CAD build for the part. Positions are in the model's coordinates, mm. Face numbers are marked on the shaded views. A direction names the side the tool comes from. Round coordinates to 2 decimals unless told otherwise and drop trailing zeros. Write each loop counter-clockwise with the first axis right and the second up, starting at its lowest first coordinate (ties: lowest second). Pieces come first, ordered by that corner, then holes. Notation, with made-up numbers: (7, 33) - (44, 33) arc R19 cw to (44, 55) - close; hole circle Ø11 at (36.25, 1). An arc over 180 degrees is marked (long way). Answer in a Markdown table with one row per item.
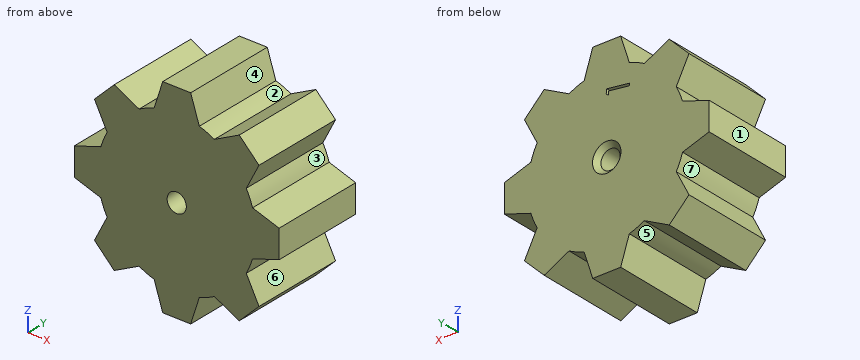
```python
from build123d import *

# Parameters (mm, degrees)
SKETCH1_R           = 1.03
BOSS_EXTRUDE1_DEPTH = 10
CUT_EXTRUDE1_DEPTH  = 1
CHAMFER1_SIZE       = 0.5


with BuildPart() as part:
    # Sketch1 → Boss-Extrude1 (new body)
    with BuildSketch(Plane(origin=(0, 0, 0), x_dir=(1, 0, 0), z_dir=(0, 1, 0))):
        with BuildLine():
            Line((-1.5, 11), (1.5, 11))
            Line((1.5, 11), (2.425924848, 8.146464793))
            ThreePointArc((2.425924848, 8.146464793), (3.252809175, 7.852976026), (4.045032587, 7.475808409))
            Line((4.045032587, 7.475808409), (6.717514421, 8.838834765))
            Line((6.717514421, 8.838834765), (8.838834765, 6.717514421))
            Line((8.838834765, 6.717514421), (7.475808409, 4.045032587))
            ThreePointArc((7.475808409, 4.045032587), (7.852976026, 3.252809175), (8.146464793, 2.425924848))
            Line((8.146464793, 2.425924848), (11, 1.5))
            Line((11, 1.5), (11, -1.5))
            Line((11, -1.5), (8.146464793, -2.425924848))
            ThreePointArc((8.146464793, -2.425924848), (7.852976026, -3.252809175), (7.475808409, -4.045032587))
            Line((7.475808409, -4.045032587), (8.838834765, -6.717514421))
            Line((8.838834765, -6.717514421), (6.717514421, -8.838834765))
            Line((6.717514421, -8.838834765), (4.045032587, -7.475808409))
            ThreePointArc((4.045032587, -7.475808409), (3.252809175, -7.852976026), (2.425924848, -8.146464793))
            Line((2.425924848, -8.146464793), (1.5, -11))
            Line((1.5, -11), (-1.5, -11))
            Line((-1.5, -11), (-2.425924848, -8.146464793))
            ThreePointArc((-2.425924848, -8.146464793), (-3.252809175, -7.852976026), (-4.045032587, -7.475808409))
            Line((-4.045032587, -7.475808409), (-6.717514421, -8.838834765))
            Line((-6.717514421, -8.838834765), (-8.838834765, -6.717514421))
            Line((-8.838834765, -6.717514421), (-7.475808409, -4.045032587))
            ThreePointArc((-7.475808409, -4.045032587), (-7.852976026, -3.252809175), (-8.146464793, -2.425924848))
            Line((-8.146464793, -2.425924848), (-11, -1.5))
            Line((-11, -1.5), (-11, 1.5))
            Line((-11, 1.5), (-8.146464793, 2.425924848))
            ThreePointArc((-8.146464793, 2.425924848), (-7.852976026, 3.252809175), (-7.475808409, 4.045032587))
            Line((-7.475808409, 4.045032587), (-8.838834765, 6.717514421))
            Line((-8.838834765, 6.717514421), (-6.717514421, 8.838834765))
            Line((-6.717514421, 8.838834765), (-4.045032587, 7.475808409))
            ThreePointArc((-4.045032587, 7.475808409), (-3.252809175, 7.852976026), (-2.425924848, 8.146464793))
            Line((-2.425924848, 8.146464793), (-1.5, 11))
        make_face()
        with Locations(Location((0, 0, 0), (0, 0, 270))):
            Circle(SKETCH1_R, mode=Mode.SUBTRACT)
    extrude(amount=BOSS_EXTRUDE1_DEPTH)

    # Sketch2 → Cut-Extrude1 (cut)
    with BuildSketch(Plane(origin=(0, 10, 0), x_dir=(1, 0, 0), z_dir=(0, 1, 0))):
        Polygon((0.061172217, -6.025718493), (-0.003431149, -6.509993333), (-2.466872655, -6.181467692), (-2.434320572, -5.936575865), (-0.212265283, -6.233050224), (-0.160682751, -5.846431634), align=None)
    extrude(amount=-CUT_EXTRUDE1_DEPTH, mode=Mode.SUBTRACT)

    # Chamfer1
    chamfer1_edges = [part.edges().sort_by_distance(p)[0] for p in [
        (0, 10, -1.03),
    ]]
    chamfer(chamfer1_edges, length=CHAMFER1_SIZE)


solid = part.part
```
Q1. Saw through at C-C on x = 6.25. List the corners of the cut face in (y, z).
Computed:
| item | result |
|---|---|
| outline | (0, -8.6) - (10, -8.6) - (10, 8.6) - (0, 8.6) - close |
Q2. Saw through at D-D on z = -7. List the corners of the cut face in (x, y).
Computed:
| item | result |
|---|---|
| outline | (-8.56, 0) - (8.56, 0) - (8.56, 10) - (-8.56, 10) - close |
Q3. Pull direction X, two halves, no side cores. Call the marked faces 1, 2 and 3: released by +X, released by -X, zero draft, split by the parting line, or undercut.
Computed:
| item | result |
|---|---|
| face 1 | released by -X |
| face 2 | undercut |
| face 3 | released by +X |
Q4. Saw through at A-A on z = 0. List the corners of the cut face in (x, y), then the cut area to 3 significant figures.
Computed:
| item | result |
|---|---|
| outline | (-11, 0) - (-1.03, 0) - (-1.03, 9.5) - (-1.53, 10) - (-11, 10) - close; (1.03, 0) - (11, 0) - (11, 10) - (1.53, 10) - (1.03, 9.5) - close |
| area | 199 mm2 |
Q5. 3-axis set-ups, long thin cutter, end or side, ignore diameter. For the marked faces 4, 5, 6 and 7: which of +Z, -Z, +X, -X, +Y, -Y reach the whole face in a straight line?
Computed:
| item | result |
|---|---|
| face 4 | +Z, +Y, -Y |
| face 5 | -Z, +Y, -Y |
| face 6 | +X, +Y, -Y |
| face 7 | -X, +Y, -Y |
Q6. Drill centre lines: line 1 (X direction, y = 6.25, z = 0); line 2 (X direction, y = 6.25, z = 8.75); line 3 (X direction, y = 5.75, z = 0.5). Where is each one in solid material? Low to high.
Computed:
| item | result |
|---|---|
| line 1 | x = -11 to -1.03, 1.03 to 11 |
| line 2 | x = -6.81 to -6.54, -2.23 to 2.23, 6.54 to 6.81 |
| line 3 | x = -11 to -0.9, 0.9 to 11 |
Q7. Flat gauge pin, fed straight in: pin 1 (1.5 mm diameter, centred on y = 7.5, z = -5.5, fed in from -X). Where does the tip first touch, or does it go through?
Computed:
| item | result |
|---|---|
| pin 1 | stops at x = -8.6 |
